Input: part model. Units: mm. Frame: model coordinates. A direction names the side the tool comes from. Coordinates: 2 decimals unless noted, no trailing zeros. Write each loop counter-clockwise with the first axis right and the second up, starting at its lowest first coordinate (ties: lowest second). Pieces come first, ordered by that corner, then holes.
1) Set-up query: faces 4 (the flat face through (-6.35, 13, 6)), 5 (the flat face through (13, 6.35, 6)), 6 (the cylindrical face through (4.822, 12.26, 11.251)), 7 (the cylindrical face through (-12.011, -4.822, 1.449)), 8 (the cylindrical face through (4.822, -12.011, 1.449)). Return all of +Z, -Z, +X, -X, +Y, -Y with unobstructed straight access to the full face (end or side cutting, diameter ignored); none if empty.
2) Section query A-A (x = 10). Output: boundary loops of the cut face in (y, z).
3) Section query D-D (z = 10). Output: boundary loops of the cut face in (x, y), then the cut area to 3 significant figures.
4) Pin query (flat end, axial travel): pin 1 Ø1.5 at (x, z) = (-1, 6) entering from +Y (3 decimals); pin 2 Ø2 at (y, z) = (-10, 6) entering from +X; pin 3 Ø3 at (x, z) = (9.5, 6.5) entering from -Y; pin 4 Ø10 at (x, y) = (6.5, -6.5) entering from +Z. Return the tip coordinate at first contact, or that it passes through.
5) Draft query along Z for faces 1 (the cylindrical face through (2.945, 9.392, 5.129)), 2 (the cylindrical face through (-4.901, 12.011, 1.528)), 3 (the cylindrical face through (12.26, 4.822, 11.251)). Return one class per face: pulls with the +Z half, pulls with the -Z half, needs draft (parallel to the pull), parting line crosses it, or undercut.
6) Line query: L1, parallel to X at y = 5, z = 6.35; L2, parallel to Z at x = 0, y = -7.25; L3, parallel to X at y = 15.25, z = 6.35. Output: solid intervals per line, ascending.
7) Section query C-C (z = 4.25). Output: boundary loops of the cut face in (x, y), then the cut area to 3 significant figures.
from build123d import *

# Parameters (mm, degrees)
F0_W     = 12.7
F0_H     = 12.7
F1_DEPTH = 12.7
F4_DEPTH = 50.8
F3_R     = 3.1877
F5_DEPTH = 76.2
F6_R     = 5.08


with BuildPart() as f1:
    # F0 (on Top) → F1 (new body)
    with BuildSketch(Plane.XY):
        with Locations((0, 12.7)):
            Rectangle(F0_W, F0_H)
        with Locations((12.7, 0)):
            Rectangle(F0_W, F0_H)
        Rectangle(F0_W, F0_H)
        with Locations((-12.7, 0)):
            Rectangle(F0_W, F0_H)
        with Locations((0, -12.7)):
            Rectangle(F0_W, F0_H)
    extrude(amount=F1_DEPTH)

    # F2 (on face) → F4 (cut)
    with BuildSketch(Plane.YZ.offset(19.05)):
        with BuildLine():
            Line((0, 3.1623), (0, 9.5377))
            ThreePointArc((0, 9.5377), (-3.1877, 6.35), (0, 3.1623))
        make_face()
        with BuildLine():
            ThreePointArc((3.1877, 6.35), (2.2540442864, 8.6040442864), (0, 9.5377))
            Line((0, 9.5377), (0, 3.1623))
            ThreePointArc((0, 3.1623), (2.2540442864, 4.0959557136), (3.1877, 6.35))
        make_face()
    extrude(amount=-F4_DEPTH, mode=Mode.SUBTRACT)

    # F3 (on face) → F5 (cut)
    with BuildSketch(Plane.XZ.offset(19.05)):
        with Locations((0, 6.35)):
            Circle(F3_R)
    extrude(amount=-F5_DEPTH, mode=Mode.SUBTRACT)

    # F6
    f6_edges = [f1.edges().sort_by_distance(p)[0] for p in [
        (-6.35, -12.7, 0),
        (6.35, -12.7, 0),
        (12.7, -6.35, 0),
        (12.7, 6.35, 0),
        (6.35, 12.7, 0),
        (-6.35, 12.7, 0),
        (-12.7, -6.35, 0),
        (-12.7, 6.35, 0),
        (-12.7, -6.35, 12.7),
        (-6.35, -12.7, 12.7),
        (12.7, -6.35, 12.7),
        (-12.7, 6.35, 12.7),
        (-6.35, 12.7, 12.7),
        (6.35, 12.7, 12.7),
        (6.35, -12.7, 12.7),
        (12.7, 6.35, 12.7),
    ]]
    fillet(f6_edges, radius=F6_R)


solid = f1.part
Answer:
1. face 4: +Z, -Z, -X, +Y
1. face 5: +Z, -Z, +X, +Y
1. face 6: +Z, +X, +Y
1. face 7: -Z, -X, -Y
1. face 8: -Z, +X, -Y
2. outline: (-6.35, 5.08) arc R5.08 ccw to (-1.27, 0) - (1.27, 0) arc R5.08 ccw to (6.35, 5.08) - (6.35, 7.62) arc R5.08 ccw to (1.27, 12.7) - (-1.27, 12.7) arc R5.08 ccw to (-6.35, 7.62) - close; hole circle Ø6.38 at (0, 6.35)
3. outline: (-19.05, -5.76) - (-5.76, -5.76) - (-5.76, -19.05) - (5.76, -19.05) - (5.76, -5.76) - (19.05, -5.76) - (19.05, 5.76) - (5.76, 5.76) - (5.76, 19.05) - (-5.76, 19.05) - (-5.76, 5.76) - (-19.05, 5.76) - close
3. area: 745 mm2
4. pin 1: passes through
4. pin 2: stops at x = 6.35
4. pin 3: stops at y = -6.35
4. pin 4: stops at z = 12.69
5. face 1: undercut
5. face 2: pulls with the -Z half
5. face 3: pulls with the +Z half
6. L1: x = -19.05 to -3.19, 3.19 to 19.05
6. L2: z = 0 to 3.16, 9.54 to 12.7
6. L3: x = -6.35 to -3.19, 3.19 to 6.35
7. outline: (-19.05, -6.28) - (-6.28, -6.28) - (-6.28, -19.05) - (-2.4, -19.05) - (-2.4, -2.4) - (-19.05, -2.4) - close; (-19.05, 2.4) - (-2.4, 2.4) - (-2.4, 19.05) - (-6.28, 19.05) - (-6.28, 6.28) - (-19.05, 6.28) - close; (2.4, -19.05) - (6.28, -19.05) - (6.28, -6.28) - (19.05, -6.28) - (19.05, -2.4) - (2.4, -2.4) - close; (2.4, 2.4) - (19.05, 2.4) - (19.05, 6.28) - (6.28, 6.28) - (6.28, 19.05) - (2.4, 19.05) - close
7. area: 457 mm2
